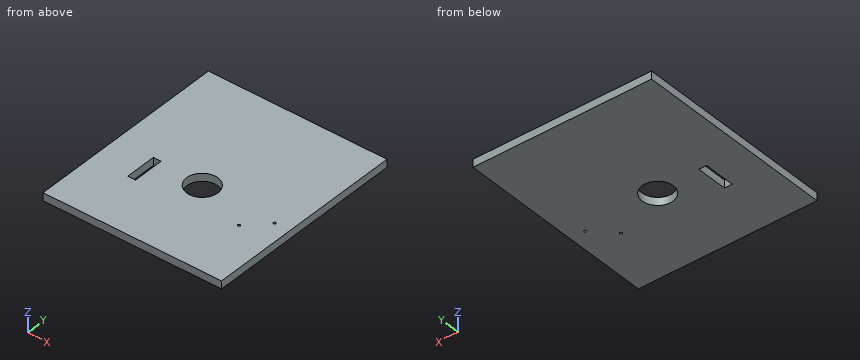
Autodesk Inventor part; units mm, degrees
ref_plane "YZ Plane" through (0, 0, 0) normal (1, 0, 0) x (0, 1, 0)
ref_plane "XZ Plane" through (0, 0, 0) normal (0, 1, 0) x (-1, 0, 0)
ref_plane "XY Plane" through (0, 0, 0) normal (0, 0, 1) x (1, 0, 0)
sketch "Sketch1" plane through (0, 0, 0) normal (0, 0, 1) x (1, 0, 0)
  line L0 (-19.7465, 14.2682) -> (107.2535, 14.2682)
  line L1 (107.2535, 14.2682) -> (107.2535, -112.7318)
  line L2 (107.2535, -112.7318) -> (-19.7465, -112.7318)
  line L3 (-19.7465, -112.7318) -> (-19.7465, 14.2682)
  point P0 (0, 0)
  dimension "d0" = 127
  dimension "d1" = 127
extrude "Extrusion1" add sketch "Sketch1" along normal blind 6.35
sketch "Sketch2" plane through (0, 0, 6.35) normal (0, 0, 1) x (1, 0, 0)
  line L0 (107.2535, -112.7318) -> (-19.7465, -112.7318)
  line L1 (-19.7465, -112.7318) -> (43.7535, -112.7318)
  line L2 (43.7535, -112.7318) -> (43.7535, -61.9318)
  line L3 (43.7535, -61.9318) -> (66.7535, -61.9318)
  line L4 (66.7535, -61.9318) -> (73.1035, -61.9318)
  line L5 (73.1035, -61.9318) -> (113.1035, -61.9318)
  line L6 (113.1035, -61.9318) -> (113.1035, -93.9318)
  line L7 (113.1035, -93.9318) -> (73.1035, -93.9318)
  line L8 (73.1035, -93.9318) -> (73.1035, -61.9318)
  point P0 (0, 0)
  dimension "d4" = 50.8
  dimension "d5" = 23
  dimension "d6" = 6.35
  dimension "d7" = 40
  dimension "d8" = 32
extrude "Extrusion2" add sketch "Sketch2" along normal blind 6.35
sketch "Sketch3" plane through (107.2535, -112.7318, 0) normal (1, 0, 0) x (0, 0, -1)
  line L0 (-6.35, 127) -> (-6.35, 50.8)
  line L1 (-6.35, 50.8) -> (-6.35, 18.8)
  line L2 (-6.35, 18.8) -> (-6.35, 0)
  line L3 (0, 0) -> (-6.35, 0)
  line L4 (0, 127) -> (0, 0)
  line L5 (0, 127) -> (-6.35, 127)
  point P0 (0, 112.7318)
extrude "Extrusion3" add sketch "Sketch3" along normal blind 12.7
sketch "Sketch4" plane through (-19.7465, -112.7318, 0) normal (-1, 0, 0) x (0, 0, 1)
  line L0 (6.35, 0) -> (6.35, 127)
  line L1 (0, 127) -> (6.35, 127)
  line L2 (0, 0) -> (0, 127)
  line L3 (0, 0) -> (6.35, 0)
  point P0 (0, 112.7318)
extrude "Extrusion4" add sketch "Sketch4" along normal blind 12.7
sketch "Sketch5" plane through (0, 0, 6.35) normal (0, 0, 1) x (1, 0, 0)
  line L0 (119.9535, -112.7318) -> (-32.4465, -112.7318)
  line L1 (119.9535, -112.7318) -> (43.7535, -112.7318)
  line L2 (43.7535, -112.7318) -> (43.7535, -61.9318)
  line L3 (43.7535, -61.9318) -> (20.7535, -61.9318)
  line L4 (20.7535, -61.9318) -> (14.4035, -61.9318)
  line L5 (14.4035, -61.9318) -> (8.0535, -61.9318)
  line L6 (8.0535, -61.9318) -> (14.4035, -61.9318)
  line L7 (14.4035, -61.9318) -> (14.4035, -87.3318)
  line L8 (14.4035, -87.3318) -> (8.0535, -87.3318)
  line L9 (8.0535, -87.3318) -> (8.0535, -61.9318)
  point P0 (0, 0)
  dimension "d15" = 23
  dimension "d16" = 6.35
  dimension "d17" = 6.35
  dimension "d18" = 25.4
extrude "Extrusion5" cut sketch "Sketch5" against normal blind 12.7
sketch "Sketch6" plane through (0, 0, 6.35) normal (0, 0, 1) x (1, 0, 0)
  line L0 (119.9535, -112.7318) -> (119.9535, 14.2682)
  line L1 (113.1035, -61.9318) -> (119.9535, -61.9318)
  line L2 (119.9535, -61.9318) -> (119.9535, -93.9318)
  line L3 (119.9535, -93.9318) -> (113.1035, -93.9318)
  line L4 (113.1035, -93.9318) -> (113.1035, -61.9318)
  point P0 (0, 0)
extrude "Extrusion6" cut sketch "Sketch6" against normal blind 12.7
sketch "Sketch7" plane through (0, 0, 12.7) normal (0, 0, 1) x (1, 0, 0)
  line L0 (73.1035, -61.9318) -> (113.1035, -61.9318)
  line L1 (73.1035, -93.9318) -> (73.1035, -61.9318)
  line L2 (113.1035, -93.9318) -> (73.1035, -93.9318)
  line L3 (113.1035, -61.9318) -> (113.1035, -93.9318)
  point P0 (0, 0)
extrude "Extrusion7" cut sketch "Sketch7" against normal blind 6.35
sketch "Sketch8" plane through (0, 0, 6.35) normal (0, 0, 1) x (1, 0, 0)
  line L0 (14.4035, -61.9318) -> (14.4035, -87.3318)
  line L1 (113.1035, -61.9318) -> (4.4035, -61.9318)
  line L2 (4.4035, -61.9318) -> (8.0535, -61.9318)
  line L3 (8.0535, -61.9318) -> (8.0535, -87.3318)
  line L4 (8.0535, -87.3318) -> (4.4035, -87.3318)
  line L5 (4.4035, -87.3318) -> (4.4035, -61.9318)
  point P0 (0, 0)
  dimension "d25" = 108.7
extrude "Extrusion8" cut sketch "Sketch8" against normal blind 6.35
sketch "Sketch9" plane through (0, 0, 6.35) normal (0, 0, 1) x (1, 0, 0)
  line L0 (4.4035, -61.9318) -> (14.4035, -61.9318)
  line L1 (14.4035, -61.9318) -> (14.4035, -87.3318)
  line L2 (14.4035, -87.3318) -> (4.4035, -87.3318)
  line L3 (4.4035, -87.3318) -> (4.4035, -61.9318)
  line L4 (4.4035, -61.9318) -> (10.7535, -61.9318)
  line L5 (10.7535, -61.9318) -> (10.7535, -87.3318)
  line L6 (10.7535, -87.3318) -> (4.4035, -87.3318)
  line L7 (4.4035, -87.3318) -> (4.4035, -61.9318)
  point P0 (0, 0)
  dimension "d28" = 6.35
extrude "Extrusion9" add sketch "Sketch9" against normal blind 6.35 contours L0 L1 L2 L5
sketch "Sketch10" plane through (0, 0, 0) normal (0, 0, -1) x (-1, 0, 0)
  line L0 (-113.1035, -61.9318) -> (-101.1035, -61.9318)
  line L1 (-101.1035, -61.9318) -> (-101.1035, -69.9318)
  line L2 (-101.1035, -69.9318) -> (-113.1035, -69.9318)
  line L3 (-113.1035, -69.9318) -> (-113.1035, -61.9318)
  line L4 (-101.1035, -69.9318) -> (-85.1035, -69.9318)
  line L5 (-85.1035, -69.9318) -> (-85.1035, -85.9318)
  line L6 (-85.1035, -85.9318) -> (-101.1035, -85.9318)
  line L7 (-101.1035, -85.9318) -> (-101.1035, -69.9318)
  circle A0 centre (-101.1035, -69.9318) radius 1
  circle A1 centre (-85.1035, -85.9318) radius 1
  point P0 (0, 0)
  dimension "d31" = 12
  dimension "d32" = 8
  dimension "d33" = 16
  dimension "d34" = 16
  dimension "d35" = 2
  dimension "d36" = 2
extrude "Extrusion10" cut sketch "Sketch10" against normal blind 6.35 contours A0 L4 L1 | L1 L2 A0 | L2 L7 A0 | L4 A0 L7 | A1 L6 L5 | L5 L6 A1
sketch "Sketch11" plane through (113.1035, -93.9318, 6.35) normal (1, 0, 0) x (0, 0, -1)
  line L0 (0, 32) -> (0, 0)
  line L1 (0, 0) -> (6.35, 0)
  line L2 (6.35, 32) -> (6.35, 0)
  line L3 (0, 32) -> (6.35, 32)
  point P0 (6.35, 93.9318)
extrude "Extrusion11" add sketch "Sketch11" along normal blind 7.62
sketch "Sketch12" plane through (119.9535, -112.7318, 0) normal (1, 0, 0) x (0, 0, -1)
  line L0 (-6.35, 50.8) -> (0, 50.8)
  line L1 (0, 50.8) -> (0, 11.311)
  line L2 (0, 11.311) -> (-6.35, 11.311)
  line L3 (-6.35, 11.311) -> (-6.35, 50.8)
  point P0 (0, 112.7318)
extrude "Extrusion12" cut sketch "Sketch12" along normal blind 7.62
sketch "Sketch13" plane through (0, 0, 0) normal (0, 0, -1) x (-1, 0, 0)
  line L0 (-10.7535, -87.3318) -> (-4.4035, -87.3318)
  line L1 (-4.4035, -87.3318) -> (-4.4035, -90.6318)
  line L2 (-4.4035, -90.6318) -> (-10.7535, -90.6318)
  line L3 (-10.7535, -90.6318) -> (-10.7535, -87.3318)
  point P0 (0, 0)
  dimension "d43" = 3.3
extrude "Extrusion13" cut sketch "Sketch13" against normal blind 7.62
sketch "Sketch14" plane through (0, 0, 0) normal (0, 0, -1) x (-1, 0, 0)
  line L0 (-4.4035, -61.9318) -> (-4.4035, -90.6318)
  line L1 (-10.7535, -61.9318) -> (-4.4035, -61.9318)
  line L2 (-4.4035, -61.9318) -> (-4.4035, -65.2318)
  line L3 (-4.4035, -65.2318) -> (-10.7535, -65.2318)
  line L4 (-10.7535, -65.2318) -> (-10.7535, -61.9318)
  point P0 (0, 0)
  dimension "d46" = 3.3
extrude "Extrusion14" add sketch "Sketch14" against normal blind 7.62
sketch "Sketch15" plane through (0, 0, 7.62) normal (0, 0, 1) x (1, 0, 0)
  line L0 (10.7535, -65.2318) -> (4.4035, -65.2318)
  line L1 (10.7535, -61.9318) -> (10.7535, -65.2318)
  line L2 (4.4035, -61.9318) -> (10.7535, -61.9318)
  line L3 (4.4035, -65.2318) -> (4.4035, -61.9318)
  point P0 (0, 0)
extrude "Extrusion15" cut sketch "Sketch15" against normal blind 1.27
sketch "Sketch16" plane through (119.9535, -112.7318, 0) normal (0, -1, 0) x (1, 0, 0)
  line L0 (0, 6.35) -> (-152.4, 6.35)
  line L1 (-152.4, 6.35) -> (-152.4, 0)
  line L2 (0, 0) -> (-152.4, 0)
  line L3 (0, 0) -> (0, 6.35)
  point P0 (-119.9535, 0)
extrude "Extrusion16" add sketch "Sketch16" along normal blind 25.4
sketch "Sketch17" plane through (119.9535, 14.2682, 6.35) normal (0, 1, 0) x (1, 0, 0)
  line L0 (-152.4, 0) -> (0, 0)
  line L1 (-152.4, 6.35) -> (0, 6.35)
  line L2 (0, 0) -> (-6.35, 0)
  line L3 (-6.35, 0) -> (-6.35, 6.35)
  line L4 (-6.35, 6.35) -> (0, 6.35)
  line L5 (0, 6.35) -> (0, 0)
  line L6 (-152.4, 6.35) -> (-146.05, 6.35)
  line L7 (-146.05, 6.35) -> (-146.05, 0)
  line L8 (-146.05, 0) -> (-152.4, 0)
  line L9 (-152.4, 0) -> (-152.4, 6.35)
  point P0 (-119.9535, 6.35)
  dimension "d53" = 6.35
  dimension "d54" = 6.35
extrude "Extrusion17" cut sketch "Sketch17" against normal blind 177.8 contours L9 L1 L7 L0 | L3 L1 L5 L0
sketch "Sketch18" plane through (0, 0, 0) normal (0, 0, -1) x (-1, 0, 0)
  line L0 (-113.6035, -138.1318) -> (26.0965, -138.1318)
  line L1 (-10.7535, -65.2318) -> (-4.4035, -65.2318)
  line L2 (-43.7535, -138.1318) -> (-43.7535, -112.7318)
  circle A0 centre (-43.7535, -112.7318) radius 12.7
  point P0 (0, 0)
  dimension "d57" = 25.4
  dimension "d58" = 25.4
extrude "Extrusion18" cut sketch "Sketch18" against normal blind 25.4
sketch "Sketch19" plane through (0, 0, 0) normal (0, 0, -1) x (-1, 0, 0)
  line L0 (-113.6035, -138.1318) -> (26.0965, -138.1318)
  line L1 (-10.7535, -65.2318) -> (-4.4035, -65.2318)
  line L2 (-43.7535, -138.1318) -> (-43.7535, -68.2818)
  circle A0 centre (-43.7535, -68.2818) radius 12.7
  point P0 (0, 0)
  dimension "d61" = 69.85
  dimension "d62" = 25.4
extrude "Extrusion19" cut sketch "Sketch19" against normal blind 25.4
sketch "Sketch20" plane through (0, 0, 0) normal (0, 0, -1) x (-1, 0, 0)
  circle A0 centre (-43.7535, -112.7318) radius 12.7
  point P0 (0, 0)
extrude "Extrusion20" add sketch "Sketch20" against normal blind 6.35
sketch "Sketch21" plane through (-26.0965, 14.2682, 6.35) normal (0, 1, 0) x (1, 0, 0)
  line L0 (0, 6.35) -> (0, 0)
  line L1 (0, 0) -> (139.7, 0)
  line L2 (139.7, 0) -> (139.7, 6.35)
  line L3 (0, 6.35) -> (139.7, 6.35)
  point P0 (26.0965, 6.35)
extrude "Extrusion21" add sketch "Sketch21" along normal blind 12.7
sketch "Sketch22" plane through (113.6035, -138.1318, 6.35) normal (1, 0, 0) x (0, 0, -1)
  line L0 (6.35, 0) -> (0, 0)
  line L1 (6.35, 165.1) -> (6.35, 0)
  line L2 (6.35, 165.1) -> (0, 165.1)
  line L3 (0, 0) -> (0, 165.1)
  point P0 (6.35, 138.1318)
extrude "Extrusion22" add sketch "Sketch22" along normal blind 3.175
sketch "Sketch23" plane through (-26.0965, -138.1318, 0) normal (-1, 0, 0) x (0, 0, 1)
  line L0 (6.35, 0) -> (0, 0)
  line L1 (6.35, 165.1) -> (6.35, 0)
  line L2 (6.35, 165.1) -> (0, 165.1)
  line L3 (0, 0) -> (0, 165.1)
  point P0 (0, 138.1318)
extrude "Extrusion23" add sketch "Sketch23" along normal blind 3.175
sketch "Sketch24" plane through (0, 0, 6.35) normal (0, 0, 1) x (1, 0, 0)
  line L0 (4.4035, -65.2318) -> (1.2285, -65.2318)
  line L1 (1.2285, -65.2318) -> (1.2285, -90.6318)
  line L2 (1.2285, -90.6318) -> (4.4035, -90.6318)
  line L3 (4.4035, -90.6318) -> (4.4035, -65.2318)
  point P0 (0, 0)
  dimension "d73" = 3.175
extrude "Extrusion24" cut sketch "Sketch24" against normal blind 6.35
sketch "Sketch25" plane through (0, 0, 6.35) normal (0, 0, 1) x (1, 0, 0)
  line L0 (10.7535, -65.2318) -> (7.5785, -65.2318)
  line L1 (7.5785, -65.2318) -> (7.5785, -91.3197)
  line L2 (7.5785, -91.3197) -> (10.7535, -91.3197)
  line L3 (10.7535, -91.3197) -> (10.7535, -65.2318)
  point P0 (0, 0)
  dimension "d76" = 3.175
extrude "Extrusion25" add sketch "Sketch25" against normal blind 6.35
sketch "Sketch26" plane through (0, 0, 0) normal (0, 0, -1) x (-1, 0, 0)
  circle A0 centre (-101.1035, -69.9318) radius 1
  circle A1 centre (-85.1035, -85.9318) radius 1
  line L0 (-1.2285, -90.6318) -> (-7.5785, -90.6318)
  line L1 (-101.1035, -69.9318) -> (-104.2785, -69.9318)
  line L2 (-85.1035, -85.9318) -> (-88.2785, -85.9318)
  circle A2 centre (-104.2785, -69.9318) radius 1
  circle A3 centre (-88.2785, -85.9318) radius 1
  point P0 (0, 0)
  dimension "d79" = 3.175
  dimension "d80" = 3.175
extrude "Extrusion26" cut sketch "Sketch26" against normal blind 6.35 contours A2 | A3
sketch "Sketch27" plane through (0, 0, 0) normal (0, 0, -1) x (-1, 0, 0)
  circle A0 centre (-101.1035, -69.9318) radius 1
  circle A1 centre (-85.1035, -85.9318) radius 1
  point P0 (0, 0)
extrude "Extrusion27" add sketch "Sketch27" against normal blind 6.35
properties part number "frontbase"
Model file for the job. Use its own axes, mm. Give positions to 0.01 mm unless a question says otherwise; leave off trailing zeros. Loops run counter-clockwise (first coordinate to the right, second up) from the corner with the lowest first, then second, coordinate; pieces in that order, holes last. Notation, with made-up numbers: (34.25, -32.5) - (46.25, -32.5) arc R27 cw to (46.25, -9.5) - close; hole circle Ø4 at (75, 4.25). An arc over 180 degrees is marked (long way). One line per item, written item: value. Start each with the question number.
1. Pin check, flat tip, straight feed: pin 1 (1.6 mm diameter, centred on x = 88.28, y = -85.93, fed in from +Z). Stop position of the tip, or through.
2. Slice it at C-C (z = 5). List the corners of the cut face in (x, y), plus the area to 3 significant figures.
3. Slice it at B-B (y = -78.5). List the corners of the cut face in (x, z).
4. Probe L1, parallel to Y at x = 46, z = 4.25; L2, parallel to Y at x = 55, z = 4; L3, parallel to X at y = -62, z = 1.25. List the from-to ranges inside material, lowest first. Write a range as from..to.
5. Slice it at A-A (x = 41). List the corners of the cut face in (y, z).
Solution:
1. pin 1: passes through
2. outline: (-29.27, -138.13) - (116.78, -138.13) - (116.78, 26.97) - (-29.27, 26.97) - close; hole (1.23, -90.63) - (7.58, -90.63) - (7.58, -65.23) - (1.23, -65.23) - close; hole circle Ø25.4 at (43.75, -68.28); hole circle Ø2 at (88.28, -85.93); hole circle Ø2 at (104.28, -69.93)
2. area: 23,400 mm^2
3. outline: (-29.27, 0) - (1.23, 0) - (1.23, 6.35) - (-29.27, 6.35) - close; (7.58, 0) - (36.21, 0) - (36.21, 6.35) - (7.58, 6.35) - close; (51.3, 0) - (116.78, 0) - (116.78, 6.35) - (51.3, 6.35) - close
4. L1: y = -138.13..-80.78, -55.78..26.97
4. L2: y = -138.13..-74.18, -62.38..26.97
4. L3: x = -29.27..32.72, 54.79..116.78
5. outline: (-138.13, 0) - (-80.68, 0) - (-80.68, 6.35) - (-138.13, 6.35) - close; (-55.88, 0) - (26.97, 0) - (26.97, 6.35) - (-55.88, 6.35) - close
